Can you work these out from the drawing? Everything is in mm from the part's minimum corner. Give positions to 0.01 mm unless a question says otherwise; leave off trailing zeros. Loops run counter-clockwise (first coordinate to the right, second up) from the corner with the lowest first, then second, coordinate; pieces in that order, holes last. Notation, with made-up numbers: (-18.75, 0) - (16.25, 0) arc R11 cw to (16.25, 11) - close; hole circle Ø1 at (81, 76.25). An arc over 180 degrees is marked (long way). Answer in a Markdown table with one row per item. Add a question column.
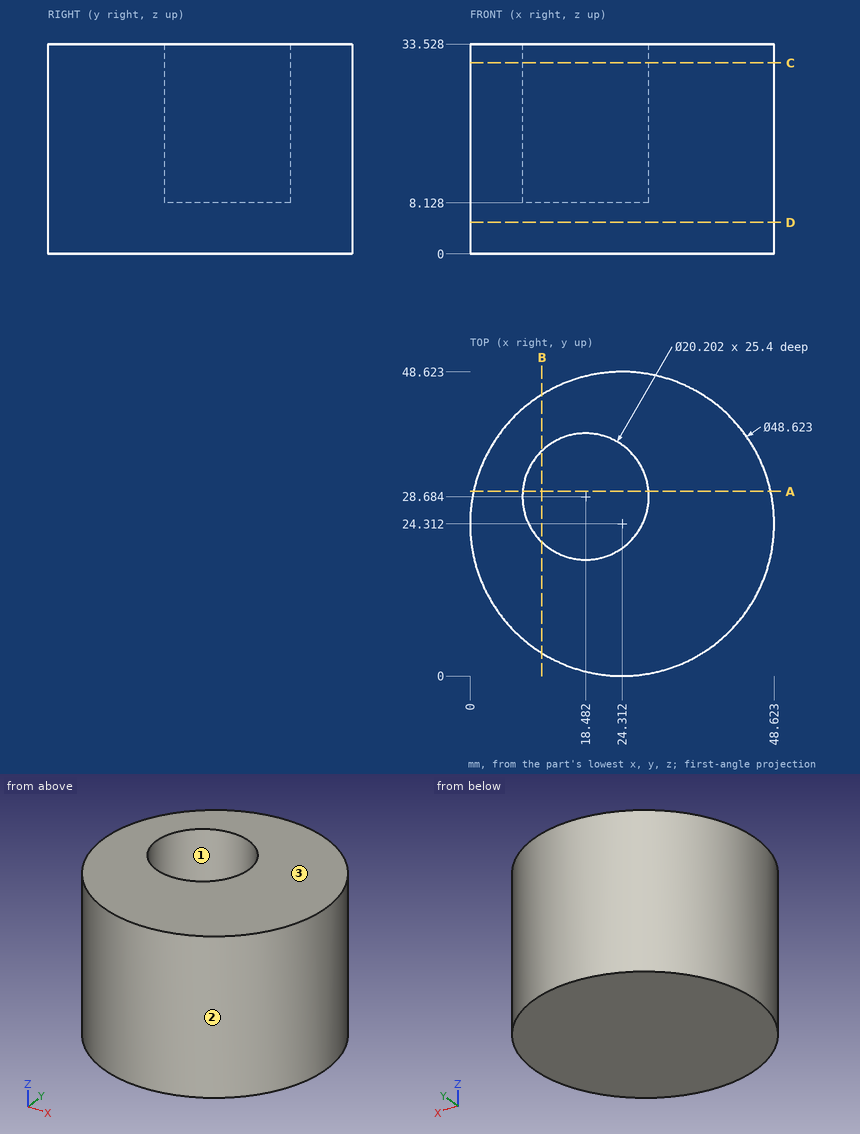
(1) I want a section at A-A on y = 29.5. Please give me the cut outline in (x, z), then the cut area to 3 significant figures.
(2) Please list where these lines run through material, in increasing order: line 1 (X direction, y = 23.5, z = 2); line 2 (Z direction, x = 21.5, y = 27); line 3 (X direction, y = 25, z = 29.5) (1 decimal).
(3) We'd pull the mould along Y, two halves only. Please class the marked faces 1, 2 and 3: pulls with the +Y half, pulls with the -Y half, needs draft (parallel to the pull), parting line crosses it, or undercut.
(4) I want a section at D-D on z = 5. Please give me the cut outline in (x, y).
(5) I want a section at C-C on z = 30.5. Please give me the cut outline in (x, y), then the cut area to 3 significant figures.
(6) I want a section at B-B on x = 11.5. Please give me the cut outline in (y, z).
(7) For pin 1 Ø12 at (x, z) = (14.5, 17) entering from +Y; pin 2 Ø1 at (y, z) = (26.5, 27.5) entering from +X; pin 3 Ø2 at (x, z) = (20, 12) entering from +Y, each with a flat end and sliding along its axis, tell me the tip position at first contact or that it passes through.
Reported:
| question | item | result |
|---|---|---|
| 1 | outline | (0.56, 0) - (48.06, 0) - (48.06, 33.53) - (28.55, 33.53) - (28.55, 8.13) - (8.41, 8.13) - (8.41, 33.53) - (0.56, 33.53) - close |
| 1 | area | 1,080 mm² |
| 2 | line 1 | 0.01 to 48.61 |
| 2 | line 2 | 0 to 8.13 |
| 2 | line 3 | 0 to 9.1, 27.9 to 48.6 |
| 3 | face 1 | undercut |
| 3 | face 2 | parting line crosses it |
| 3 | face 3 | needs draft |
| 4 | outline | circle Ø48.62 at (24.31, 24.31) |
| 5 | outline | circle Ø48.62 at (24.31, 24.31); hole circle Ø20.2 at (18.48, 28.68) |
| 5 | area | 1,540 mm² |
| 6 | outline | (3.65, 0) - (44.97, 0) - (44.97, 33.53) - (35.98, 33.53) - (35.98, 8.13) - (21.38, 8.13) - (21.38, 33.53) - (3.65, 33.53) - close |
| 7 | pin 1 | y = 48.32 |
| 7 | pin 2 | x = 48.56 |
| 7 | pin 3 | y = 48.4 |
